Model file for the job. Use its own axes, mm. Face numbers are marked on the shaded views. A direction names the side the tool comes from. Coordinates: 2 decimals unless noted, no trailing zeros. Loops run counter-clockwise (first coordinate to the right, second up) from the corner with the lowest first, then second, coordinate; pieces in that order, holes last. Notation, with made-up numbers: (53.25, 83.5) -> (78.25, 83.5) arc R10 ccw to (78.25, 98.5) -> close; hole circle Ø11 at (-11, 68.25). An arc over 180 degrees is marked (long way). Use one line per item in the form item = value.
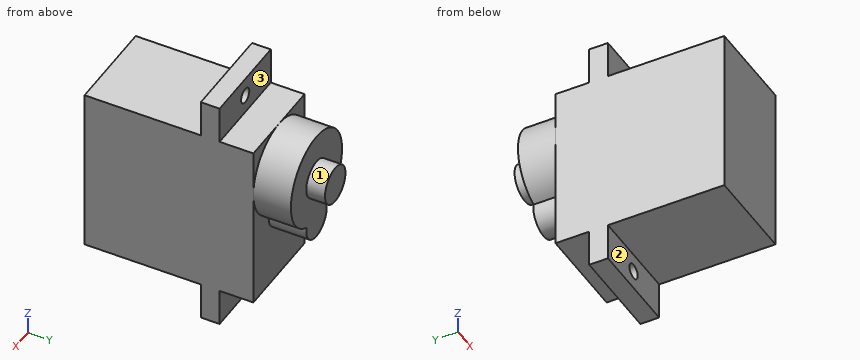
```python
from build123d import *

# Parameters (mm, degrees)
SKETCH1_W                = 12.5
SKETCH1_H                = 22.5
BOSS_EXTRUDE1_DEPTH      = 22.5
BOSS_EXTRUDE2_DEPTH      = 5
BOSS_EXTRUDE2_DEPTH_BACK = 27.5
SKETCH2_W                = 12.5
SKETCH2_H                = 2.5
BOSS_EXTRUDE3_DEPTH      = 5
SKETCH4_R                = 2.5
BOSS_EXTRUDE4_DEPTH      = 2.5
SKETCH5_R                = 1
CUT_EXTRUDE1_DEPTH       = 36.163901945


with BuildPart() as part:
    # Sketch1 → Boss-Extrude1 (new body)
    with BuildSketch(Plane.XY):
        with Locations((6.25, 11.25)):
            Rectangle(SKETCH1_W, SKETCH1_H)
    extrude(amount=BOSS_EXTRUDE1_DEPTH)

    # Sketch2 → Boss-Extrude2 (add, two sides: drawn at the far end of the back side and taken through both)
    with BuildSketch(Plane.XY.offset(22.5).offset(-BOSS_EXTRUDE2_DEPTH_BACK)):
        with Locations((6.25, 16.75)):
            Rectangle(SKETCH2_W, SKETCH2_H)
    extrude(amount=BOSS_EXTRUDE2_DEPTH + BOSS_EXTRUDE2_DEPTH_BACK)

    # Sketch3 → Boss-Extrude3 (add)
    with BuildSketch(Plane(origin=(0, 22.5, 0), x_dir=(1, 0, 0), z_dir=(0, 1, 0))):
        with BuildLine():
            ThreePointArc((3.800510257, -10.5), (6.25, -22.5), (8.699489743, -10.5))
            ThreePointArc((8.699489743, -10.5), (6.25, -7.5), (3.800510257, -10.5))
        make_face()
    extrude(amount=BOSS_EXTRUDE3_DEPTH)

    # Sketch4 → Boss-Extrude4 (add)
    with BuildSketch(Plane(origin=(0, 27.5, 0), x_dir=(1, 0, 0), z_dir=(0, 1, 0))):
        with Locations(Location((6.25, -16.25, 0), (0, 0, 270))):
            Circle(SKETCH4_R)
    extrude(amount=BOSS_EXTRUDE4_DEPTH)

    # Sketch5 → Cut-Extrude1 (cut, through all)
    with BuildSketch(Plane(origin=(0, 18, 0), x_dir=(1, 0, 0), z_dir=(0, 1, 0))):
        with Locations(Location((6.25, -25, 0), (0, 0, 270))):
            Circle(SKETCH5_R)
        with Locations(Location((6.25, 2.5, 0), (0, 0, 270))):
            Circle(SKETCH5_R)
    extrude(amount=-CUT_EXTRUDE1_DEPTH, mode=Mode.SUBTRACT)


solid = part.part
```
Q1. Band-saw the part on A-A, the plane z = 25. Write the cut outline in (x, y).
Result:
outline = (0, 15.5) -> (5.25, 15.5) -> (5.25, 18) -> (0, 18) -> close; (7.25, 15.5) -> (12.5, 15.5) -> (12.5, 18) -> (7.25, 18) -> close
Q2. Which spindle directions (+Z, -Z, +X, -X, +Y, -Y) get a long thin tool onto all of the face, cutting with end or side? Do the marked faces 1, 2 and 3. Say none if no direction does.
Result:
face_1 = +Y
face_2 = -Z, +X, -X, -Y
face_3 = +Z, +X, -X, +Y
Q3. Pin check, flat tips, straight feed: pin 1 Ø1.6 at (x, z) = (6.25, 25) entering from -Y; pin 2 Ø4 at (x, z) = (4.5, 8.5) entering from +Y; pin 3 Ø1.5 at (x, z) = (8.5, -3.5) entering from +Y; pin 4 Ø2.5 at (x, z) = (8, -1.5) entering from -Y. Stop position of each tip, or through.
Result:
pin_1 = through
pin_2 = 27.5
pin_3 = 18
pin_4 = 15.5
Q4. Band-saw the part on B-B, the plane z = 10. Write the cut outline in (x, y), and give its area (3 significant figures).
Result:
outline = (0, 0) -> (12.5, 0) -> (12.5, 22.5) -> (8.75, 22.5) -> (8.75, 27.5) -> (3.75, 27.5) -> (3.75, 22.5) -> (0, 22.5) -> close
area = 306 mm2
Q5. Wall check: line 1 along X through (y, z) = (17, 25); line 2 along Y through (x, z) = (1.5, 23); line 3 along Y through (x, z) = (10.25, 11). Give the ranges that are in metal, low to high.
Result:
line_1 = 0 to 5.25, 7.25 to 12.5
line_2 = 15.5 to 18
line_3 = 0 to 22.5
Q6. Band-saw the part on C-C, the plane x = 8.25. Write the cut outline in (y, z), and give its area (3 significant figures).
Result:
outline = (0, 0) -> (15.5, 0) -> (15.5, -5) -> (18, -5) -> (18, 0) -> (22.5, 0) -> (22.5, 8.5) -> (27.5, 8.5) -> (27.5, 14.75) -> (30, 14.75) -> (30, 17.75) -> (27.5, 17.75) -> (27.5, 22.17) -> (22.5, 22.17) -> (22.5, 22.5) -> (18, 22.5) -> (18, 27.5) -> (15.5, 27.5) -> (15.5, 22.5) -> (0, 22.5) -> close
area = 607 mm2
Q7. Band-saw the part on D-D, the plane y = 6.5. Write the cut outline in (x, z).
Result:
outline = (0, 0) -> (12.5, 0) -> (12.5, 22.5) -> (0, 22.5) -> close
